from build123d import *

# Parameters (mm, degrees)
BOSS_EXTRU_1_DEPTH      = 4
ESQUISSE2_R             = 5.05
ENL_V_MAT_EXTRU_1_DEPTH = 10
CONG_1_R                = 10


with BuildPart() as part:
    # Esquisse1 → Boss.-Extru.1 (new body)
    with BuildSketch(Plane(origin=(0, 0, 0), x_dir=(0, 0, -1), z_dir=(1, 0, 0))):
        with BuildLine():
            ThreePointArc((33.755002002, 5), (48, 0), (33.755002002, -5))
            Line((33.755002002, -5), (-33.755002002, -5))
            ThreePointArc((-33.755002002, -5), (-48, 0), (-33.755002002, 5))
            Line((-33.755002002, 5), (33.755002002, 5))
        make_face()
    extrude(amount=BOSS_EXTRU_1_DEPTH)

    # Esquisse2 → Enlèv. mat.-Extru.1 (cut)
    with BuildSketch(Plane(origin=(4, 0, 0), x_dir=(0, 0, -1), z_dir=(1, 0, 0))):
        with Locations((-40, 0)):
            Circle(ESQUISSE2_R)
        with Locations((40, 0)):
            Circle(ESQUISSE2_R)
    extrude(amount=-ENL_V_MAT_EXTRU_1_DEPTH, mode=Mode.SUBTRACT)

    # Congé1
    cong_1_edges = [part.edges().sort_by_distance(p)[0] for p in [
        (2, -5, 33.755002002),
        (2, 5, 33.755002002),
        (2, 5, -33.755002002),
        (2, -5, -33.755002002),
    ]]
    fillet(cong_1_edges, radius=CONG_1_R)


solid = part.part
CAD build for the part. Positions are in the model's coordinates, mm. A direction names the side the tool comes from. Give positions to 0.01 mm unless a question says otherwise; leave off trailing zeros. Write each loop counter-clockwise with the first axis right and the second up, starting at its lowest first coordinate (ties: lowest second). Pieces come first, ordered by that corner, then holes. Notation, with made-up numbers: M 85,81.25 L 90,81.25 A12 cw 90,86.25 Z; hole C -21,-20 d6. An arc over 180 degrees is marked long. Put each result on its own line as item: value. Start each with the question number.
(1) Band-saw the part on D-D, the plane z = 27.5. Write the cut outline in (x, y).
(2) Flat gauge pins, fed straight in: pin 1 Ø1 at (x, y) = (3, 5) entering from -Z; pin 2 Ø2 at (x, z) = (2, -14) entering from +Y; pin 3 Ø1.2 at (x, z) = (1.5, 11.5) entering from -Y. Where does each tip first touch, or does it go through?
(3) Band-saw the part on C-C, the plane x = 1.65. Write the cut outline in (y, z), and give its area (3 significant figures).
(4) Mould opens along Y. For faces 1 (the face through (2.028, 0.222, 45.045)), 2 (the face through (2.03, -5.44, -32.98)), 3 (the face through (4, 0, -1)) say: +Y half, -Y half, draft (parallel to the pull), parting line (faces both ways), or undercut.
(5) Band-saw the part on A-A, the plane y = 0. Write the cut outline in (x, z), and give its area (3 significant figures).
(6) Band-saw the part on B-B, the plane z = 40. Write the cut outline in (x, y), and give its area (3 significant figures).
(7) Probe L1, parallel to Y at x = 1.9, z = -40; L2, parallel to Z at x = 2.7, y = -1.75; L3, parallel to Y at x = 2.1, z = -0.5. List the from-to ranges inside material, lowest first.
(8) Which spindle directions (+Z, -Z, +X, -X, +Y, -Y) get a long thin tool onto all of the face, cutting with end or side? Do faces 4 (the face through (2, 5, 0)), 5 (the face through (2, 0, -48)), 6 (the face through (2, -5, 0)). Say none if no direction does.
Response values:
1. outline: M 0,-5 L 4,-5 L 4,5 L 0,5 Z
2. pin 1: stops at z = -46.61
2. pin 2: stops at y = 5
2. pin 3: stops at y = -5
3. outline: M -6.67,-35.58 A8 ccw long 6.67,-35.58 A10 cw 5,-30.05 L 5,30.05 A10 cw 6.67,35.58 A8 ccw long -6.67,35.58 A10 cw -5,30.05 L -5,-30.05 A10 cw Z; hole C 0,-40 d10.1; hole C 0,40 d10.1
3. area: 898 mm2
4. face 1: undercut
4. face 2: -Y half
4. face 3: draft
5. outline: M 0,-48 L 4,-48 L 4,-45.05 L 0,-45.05 Z; M 0,-34.95 L 4,-34.95 L 4,34.95 L 0,34.95 Z; M 0,45.05 L 4,45.05 L 4,48 L 0,48 Z
5. area: 303 mm2
6. outline: M 0,-8 L 4,-8 L 4,-5.05 L 0,-5.05 Z; M 0,5.05 L 4,5.05 L 4,8 L 0,8 Z
6. area: 23.6 mm2
7. L1: y = -8 to -5.05, 5.05 to 8
7. L2: z = -47.81 to -44.74, -35.26 to 35.26, 44.74 to 47.81
7. L3: y = -5 to 5
8. face 4: +X, -X, +Y
8. face 5: +X, -X
8. face 6: +X, -X, -Y
